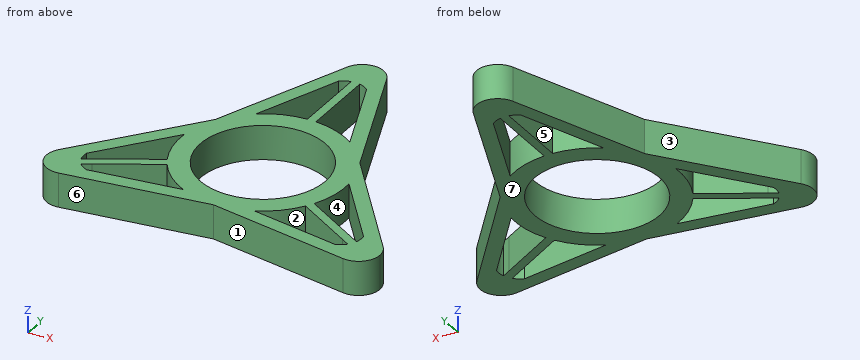
```python
from build123d import *

# Parameters (mm, degrees)
F0_R     = 11
F1_DEPTH = 6


with BuildPart() as f1:
    # F0 (on Top) → F1 (new body)
    with BuildSketch(Plane.XY):
        with BuildLine():
            Line((-23.441037, -14.399715), (-21.990769, -13.562402))
            ThreePointArc((-21.990769, -13.562402), (-22.300154, -12.875), (-22.740769, -12.263364))
            Line((-22.740769, -12.263364), (-24.191037, -13.100677))
            ThreePointArc((-24.191037, -13.100677), (-24.375767, -12.162283), (-24.317114, -11.207679))
            ThreePointArc((-24.317114, -11.207679), (-26.5881, -11.1472), (-28.47727, -12.408973))
            ThreePointArc((-28.47727, -12.408973), (-28.795345, -16.625), (-24.98512, -18.457553))
            ThreePointArc((-24.98512, -18.457553), (-22.947808, -17.45237), (-21.864692, -15.455399))
            ThreePointArc((-21.864692, -15.455399), (-22.720729, -15.028892), (-23.441037, -14.399715))
        make_face()
        with BuildLine():
            Line((-21.990769, -13.562402), (-12.165559, -7.889814))
            ThreePointArc((-12.165559, -7.889814), (-9.565708, -10.89712), (-6.246866, -13.085361))
            Line((-6.246866, -13.085361), (-21.864692, -15.455399))
            ThreePointArc((-21.864692, -15.455399), (-22.947808, -17.45237), (-24.98512, -18.457553))
            Line((-24.98512, -18.457553), (0, -14.666008))
            Line((0, -14.666008), (24.98512, -18.457553))
            ThreePointArc((24.98512, -18.457553), (22.947808, -17.45237), (21.864692, -15.455399))
            Line((21.864692, -15.455399), (6.246866, -13.085361))
            ThreePointArc((6.246866, -13.085361), (9.565708, -10.89712), (12.165559, -7.889814))
            Line((12.165559, -7.889814), (21.990769, -13.562402))
            ThreePointArc((21.990769, -13.562402), (22.300154, -12.875), (22.740769, -12.263364))
            Line((22.740769, -12.263364), (12.915559, -6.590776))
            ThreePointArc((12.915559, -6.590776), (14.220037, -2.835586), (14.455688, 1.132736))
            Line((14.455688, 1.132736), (24.317114, -11.207679))
            ThreePointArc((24.317114, -11.207679), (26.5881, -11.1472), (28.47727, -12.408973))
            Line((28.47727, -12.408973), (12.701135, 7.333004))
            Line((12.701135, 7.333004), (3.49215, 30.866525))
            ThreePointArc((3.49215, 30.866525), (0, 33.25), (-3.49215, 30.866525))
            Line((-3.49215, 30.866525), (-12.701135, 7.333004))
            Line((-12.701135, 7.333004), (-28.47727, -12.408973))
            ThreePointArc((-28.47727, -12.408973), (-26.5881, -11.1472), (-24.317114, -11.207679))
            Line((-24.317114, -11.207679), (-14.455688, 1.132736))
            ThreePointArc((-14.455688, 1.132736), (-14.201564, -2.831903), (-12.915559, -6.590776))
            Line((-12.915559, -6.590776), (-22.740769, -12.263364))
            ThreePointArc((-22.740769, -12.263364), (-22.300154, -12.875), (-21.990769, -13.562402))
        make_face()
        Circle(F0_R, mode=Mode.SUBTRACT)
        with BuildLine():
            Line((-8.208822, 11.952625), (-2.452422, 26.663078))
            ThreePointArc((-2.452422, 26.663078), (-1.655038, 27.191175), (-0.75, 27.500391))
            Line((-0.75, 27.500391), (-0.75, 14.48059))
            ThreePointArc((-0.75, 14.48059), (-4.654329, 13.732706), (-8.208822, 11.952625))
        make_face(mode=Mode.SUBTRACT)
        with BuildLine():
            ThreePointArc((0.75, 27.500391), (1.655038, 27.191175), (2.452422, 26.663078))
            Line((2.452422, 26.663078), (8.208822, 11.952625))
            ThreePointArc((8.208822, 11.952625), (4.648282, 13.714866), (0.75, 14.48059))
            Line((0.75, 14.48059), (0.75, 27.500391))
        make_face(mode=Mode.SUBTRACT)
        with BuildLine():
            ThreePointArc((21.864692, -15.455399), (22.947808, -17.45237), (24.98512, -18.457553))
            ThreePointArc((24.98512, -18.457553), (27.992401, -17.593621), (29.297749, -14.75))
            ThreePointArc((29.297749, -14.75), (29.08669, -13.509678), (28.47727, -12.408973))
            ThreePointArc((28.47727, -12.408973), (26.5881, -11.1472), (24.317114, -11.207679))
            ThreePointArc((24.317114, -11.207679), (24.375767, -12.162283), (24.191037, -13.100677))
            Line((24.191037, -13.100677), (22.740769, -12.263364))
            ThreePointArc((22.740769, -12.263364), (22.300154, -12.875), (21.990769, -13.562402))
            Line((21.990769, -13.562402), (23.441037, -14.399715))
            ThreePointArc((23.441037, -14.399715), (22.720729, -15.028892), (21.864692, -15.455399))
        make_face()
    extrude(amount=F1_DEPTH)


solid = f1.part
```
Check sheet for the modelled part. Datum: model origin and axes. Units: mm. Face numbers are marked on the shaded views. A direction names the side the tool comes from. Give positions to 0.01 mm unless a question says otherwise; leave off trailing zeros. Write each loop counter-clockwise with the first axis right and the second up, starting at its lowest first coordinate (ties: lowest second). Pieces come first, ordered by that corner, then holes. Notation, with made-up numbers: (71.25, 54) -> (99.25, 54) arc R37 cw to (99.25, 92) -> close; hole circle Ø11 at (23.5, 64.25). An arc over 180 degrees is marked (long way). Use CSV: the item, a comma, the result in double quotes. Start each with the question number.
Q1. Release check for a two-part mould opening along Y. For the marked faces 1, 2, 3 and 4 record: +Y half, -Y half, draft (parallel to the pull), parting line (faces both ways), or undercut.
Q2. Cross-section at D-D on y = 8.5. Enter the section's corners in (x, z), and give its area (3 significant figures).
Q3. Depth check by flat-ended pin: P1, Ø3, axis at y = 16.5, z = 5, coming from the -X side; P2, Ø5, axis at x = 18, y = 3, coming from the -Z side; P3, Ø2, axis at y = 25, z = 4, coming from the -X side; P4, Ø1, axis at x = 3, z = 4.5, coming from the +Y side. Enter the tip coordinate at first touch or a pass-through.
Q4. Cross-section at C-C on z = 1.45. Count the separate pieces of the cut face and the enclosed holes in it, and give its area (3 significant figures).
Q5. Scan lines: line 1 along X through (y, z) = (23.5, 3.65); line 2 along X through (y, z) = (19.5, 4.8); line 3 along X through (y, z) = (0.5, 3.2). Record each from-to range of solid material in increasing order.
Q6. Tool access check on the marked faces 5, 6 and 7. Record the directions out of +Z, -Z, +X, -X, +Y, -Y that give a thin tool (end or side, any length) a straight path to the whole face; none if there is none.
Q7. Cross-section at A-A on y = 2.5. Enter the section's corners in (x, z).
Q8. Cross-section at B-B on y = 16. Enter the section's corners in (x, z).
Working result:
1,face 1,"-Y half"
1,face 2,"undercut"
1,face 3,"+Y half"
1,face 4,"undercut"
2,outline,"(-12.24, 0) -> (-6.98, 0) -> (-6.98, 6) -> (-12.24, 6) -> close; (6.98, 0) -> (12.24, 0) -> (12.24, 6) -> (6.98, 6) -> close"
2,area,"63.1 mm^2"
3,P1,"stops at x = -9.7"
3,P2,"stops at z = 0"
3,P3,"stops at x = -6.18"
3,P4,"stops at y = 32.3"
4,separate pieces,"1"
4,enclosed holes,"7"
4,area,"743 mm^2"
5,line 1,"x = -6.37 to -3.69, -0.75 to 0.75, 3.69 to 6.37"
5,line 2,"x = -7.94 to -5.26, -0.75 to 0.75, 5.26 to 7.94"
5,line 3,"x = -18.16 to -14.96, -14.49 to -10.99, 10.99 to 14.49, 14.96 to 18.16"
6,face 5,"+Z, -Z"
6,face 6,"+Z, -Z, -Y"
6,face 7,"-Z, +X, -X, +Y, -Y"
7,outline,"(-16.56, 0) -> (-10.71, 0) -> (-10.71, 6) -> (-16.56, 6) -> close; (10.71, 0) -> (16.56, 0) -> (16.56, 6) -> (10.71, 6) -> close"
8,outline,"(-9.31, 0) -> (-6.63, 0) -> (-6.63, 6) -> (-9.31, 6) -> close; (-0.75, 0) -> (0.75, 0) -> (0.75, 6) -> (-0.75, 6) -> close; (6.63, 0) -> (9.31, 0) -> (9.31, 6) -> (6.63, 6) -> close"
